Part model, mm, in its own coordinate system. Face numbers are marked on the shaded views. A direction names the side the tool comes from. Give positions to 0.01 mm unless a question says otherwise; leave off trailing zeros. Order: outer loops, then holes, each group sorted by start corner. A loop starts at its lowest first (then second) coordinate and runs counter-clockwise, first axis right, second up. Notation, with made-up numbers: M 56,46.5 L 110,46.5 A26 ccw 110,76.5 Z; hole C 60,43.25 d1. An arc over 180 degrees is marked long. Write each question's results on one line, items separated by ' | '. Start each with the question number.
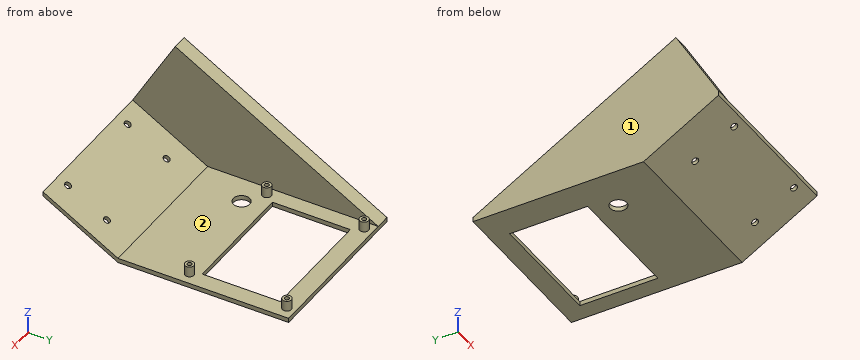
from build123d import *

# Parameters (mm, degrees)
SKETCH1_W           = 102
SKETCH1_H           = 113.73
SKETCH1_R           = 3
SKETCH1_R_2         = 5.5
SKETCH1_W_2         = 79.8
SKETCH1_H_2         = 52
BOSS_EXTRUDE1_DEPTH = 3
SKETCH1_3_R         = 3
BOSS_EXTRUDE2_DEPTH = 10
SKETCH2_R           = 1.5
CUT_EXTRUDE1_DEPTH  = 7
BOSS_EXTRUDE3_DEPTH = 102
SKETCH4_R           = 2.25
CUT_EXTRUDE2_DEPTH  = 155.667120928
BOSS_EXTRUDE4_DEPTH = 10


with BuildPart() as part:
    # Sketch1 → Boss-Extrude1 (new body)
    with BuildSketch(Plane.XY):
        with Locations((51, 56.865)):
            Rectangle(SKETCH1_W, SKETCH1_H)
        with Locations((6.05, 42.97)):
            Circle(SKETCH1_R, mode=Mode.SUBTRACT)
        with Locations((93.95, 42.97)):
            Circle(SKETCH1_R, mode=Mode.SUBTRACT)
        with Locations((18.9, 33.699)):
            Circle(SKETCH1_R_2, mode=Mode.SUBTRACT)
        with Locations((50.6, 75.42)):
            Rectangle(SKETCH1_W_2, SKETCH1_H_2, mode=Mode.SUBTRACT)
    extrude(amount=BOSS_EXTRUDE1_DEPTH)

    # Sketch1<3> → Boss-Extrude2 (add)
    with BuildSketch(Plane.XY):
        with Locations((6.05, 107.87)):
            Circle(SKETCH1_3_R)
        with Locations((93.95, 107.87)):
            Circle(SKETCH1_3_R)
        with Locations((6.05, 42.97)):
            Circle(SKETCH1_3_R)
        with Locations((93.95, 42.97)):
            Circle(SKETCH1_3_R)
    extrude(amount=BOSS_EXTRUDE2_DEPTH)

    # Sketch2 → Cut-Extrude1 (cut)
    with BuildSketch(Plane.XY.offset(10)):
        with Locations((6.05, 107.87)):
            Circle(SKETCH2_R)
        with Locations((93.95, 107.87)):
            Circle(SKETCH2_R)
        with Locations((93.95, 42.97)):
            Circle(SKETCH2_R)
        with Locations((6.05, 42.97)):
            Circle(SKETCH2_R)
    extrude(amount=-CUT_EXTRUDE1_DEPTH, mode=Mode.SUBTRACT)

    # Sketch3 → Boss-Extrude3 (add)
    with BuildSketch(Plane(origin=(102, 0, 0), x_dir=(0, 0, -1), z_dir=(1, 0, 0))):
        Polygon((-3, 0), (-31.867513459, -50), (-28.867513459, -50), (0, 0), align=None)
    extrude(amount=-BOSS_EXTRUDE3_DEPTH)

    # Sketch4 → Cut-Extrude2 (cut, through all)
    with BuildSketch(Plane(origin=(0, 1.299038106, 2.25), x_dir=(1, 0, 0), z_dir=(0, 0.4999999999999944, 0.8660254037844419))):
        with Locations(Location((17, -21.5, 0), (0, 0, 270))):
            Circle(SKETCH4_R)
        with Locations(Location((85, -21.5, 0), (0, 0, 270))):
            Circle(SKETCH4_R)
        with Locations(Location((85, -51.5, 0), (0, 0, 90))):
            Circle(SKETCH4_R)
        with Locations(Location((17, -51.5, 0), (0, 0, 90))):
            Circle(SKETCH4_R)
    extrude(amount=-CUT_EXTRUDE2_DEPTH, mode=Mode.SUBTRACT)

    # Sketch5 → Boss-Extrude4 (add)
    with BuildSketch(Plane.ZY):
        Polygon((31.867513459, -50), (81.114048046, -21.5675), (3, 113.73), (0, 113.73), (0, 0), (28.867513459, -50), align=None)
    extrude(amount=BOSS_EXTRUDE4_DEPTH)


solid = part.part
(1) Saw through at C-C on z = 34. Give the cut face in (x, y).
(2) Saw through at D-D on z = 53.5. Give the cut face in (x, y), plus the area to 3 significant figures.
(3) Probe L1, parallel to X at y = 107.87, z = 6; L2, parallel to X at y = 107.87, z = 8; L3, parallel to Y at x = 93.95, z = 7.75. List the from-to ranges inside material, lowest first.
(4) Saw through at B-B on y = -31.5. Give the cut face in (x, z), plus the area to 3 significant figures.
(5) Saw through at A-A on x = 52.5. Give the cut face in (y, z).
(6) Drop flat-ended pins along their axis: P1, Ø6.5, axis at x = 95, y = 106.5, coming from the +Z side; P2, Ø1.5, axis at x = 93.5, y = 107.5, coming from the +Z side; P3, Ø5, axis at x = 75, z = 19.5, coming from the -Y side; P4, Ø10, axis at x = 88.5, z = 38, coming from the +Y side. Give the stop position or say it passes through.
(7) Tool access for the marked faces 1 and 2: list every direction of +Z, -Z, +X, -X, +Y, -Y with a clear straight run to the whole face (end or side of a thin tool).
Taken from the geometry:
1) outline: M -10,-48.77 L 0,-48.77 L 0,60.04 L -10,60.04 Z
2) outline: M -10,-37.51 L 0,-37.51 L 0,26.26 L -10,26.26 Z | area: 638 mm²
3) L1: x = -10 to 0, 3.05 to 4.55, 7.55 to 9.05, 90.95 to 92.45, 95.45 to 96.95 | L2: x = 3.05 to 4.55, 7.55 to 9.05, 90.95 to 92.45, 95.45 to 96.95 | L3: y = -13.42 to -8.23, 39.97 to 41.47, 44.47 to 45.97, 104.87 to 106.37, 109.37 to 110.87
4) outline: M -10,18.19 L 102,18.19 L 102,21.19 L 0,21.19 L 0,63.91 L -10,63.91 Z | area: 763 mm²
5) outline: M -50,28.87 L 0,0 L 49.42,0 L 49.42,3 L 0,3 L -50,31.87 Z; M 101.42,0 L 113.73,0 L 113.73,3 L 101.42,3 Z
6) P1: stops at z = 10 | P2: stops at z = 3 | P3: stops at y = -38.11 | P4: passes through
7) face 1: +Z, -Z, -X, +Y, -Y | face 2: +Z
